Input: part model. Units: mm. Frame: model coordinates. A direction names the side the tool comes from. Coordinates: 2 decimals unless noted, no trailing zeros. Order: outer loops, then holes, each group sorted by start corner. A loop starts at its lowest first (then second) coordinate and runs counter-clockwise, first axis right, second up.
Autodesk Inventor part; units mm, degrees
ref_plane "YZ Plane" through (0, 0, 0) normal (1, 0, 0) x (0, 1, 0)
ref_plane "XZ Plane" through (0, 0, 0) normal (0, 1, 0) x (-1, 0, 0)
ref_plane "XY Plane" through (0, 0, 0) normal (0, 0, 1) x (1, 0, 0)
sketch "Sketch1" plane through (0, 0, 0) normal (0, 0, 1) x (1, 0, 0)
  line L0 (-20, 31) -> (20, 31)
  line L1 (20, 31) -> (20, 0)
  line L2 (-20, 0) -> (-20, 31)
  line L3 (40, 0) -> (40, -20)
  line L4 (40, -20) -> (-40, -20)
  line L5 (-40, -20) -> (-40, 0)
  line L6 (-40, 0) -> (-20, 0)
  line L7 (20, 0) -> (40, 0)
  circle A0 centre (0, 11) radius 9.125
  point P0 (0, 0)
  point P1 (0, 31)
  point P2 (0, -20)
  dimension "d0" = 80
  dimension "d1" = 20
  dimension "d2" = 40
  dimension "d3" = 31
  dimension "d6" = 18.25
  dimension "d7" = 20
extrude "Extrusion1" add sketch "Sketch1" along normal blind 6.5 contours L0 L1 L7 L3 L4 L5 L6 L2 | A0
sketch "Sketch2" plane through (0, 0, 6.5) normal (0, 0, 1) x (1, 0, 0)
  circle A0 centre (0, 11) radius 9.125
  line L0 (20, 31) -> (-20, 31)
  point P0 (0, 0)
  dimension "d8" = 20
  dimension "d9" = 18.25
sketch "Sketch3" plane through (0, 0, 0) normal (0, 0, -1) x (-1, 0, 0)
  line L0 (-20, 31) -> (20, 31)
  line L1 (40, -20) -> (-40, -20)
  line L2 (20, 31) -> (-20, 31)
  line L3 (-20, 31) -> (-20, -20)
  line L4 (-20, -20) -> (20, -20)
  line L5 (20, -20) -> (20, 31)
  point P0 (0, 0)
  point P1 (-20, 5.5)
  point P2 (-20, 0)
extrude "Extrusion2" add sketch "Sketch3" along normal blind 3.5
sketch "Sketch4" plane through (0, 0, -3.5) normal (0, 0, -1) x (-1, 0, 0)
  line L0 (-20, 31) -> (20, 31)
  line L1 (-20, -20) -> (20, -20)
  line L2 (11.85, 31) -> (-11.85, 31)
  line L3 (-11.85, 31) -> (-11.85, -20)
  line L4 (-11.85, -20) -> (11.85, -20)
  line L5 (11.85, -20) -> (11.85, 31)
  point P0 (0, 0)
  point P1 (0, 31)
  dimension "d12" = 23.7
extrude "Extrusion3" add sketch "Sketch4" along normal blind 5
extrude "Extrusion4" cut sketch "Sketch2" against normal up to next
fillet "Fillet1" radius 8 6 edges at (-20, 31, 1.5) (-40, 0, 3.25) (20, 31, 1.5) (-20, 0, 3.25) (40, 0, 3.25) (20, 0, 3.25)
sketch "Sketch5" plane through (0, 0, 0) normal (0, 0, -1) x (-1, 0, 0)
  arc A0 (27.9, -14) -> (32.1, -14) centre (30, -14) ccw
  arc A1 (32.1, -7.88) -> (27.9, -7.88) centre (30, -7.88) ccw
  line L0 (32.1, -7.88) -> (32.1, -14)
  line L1 (27.9, -7.88) -> (27.9, -14)
  line L2 (40, -20) -> (40, -8)
  line L3 (20, -20) -> (40, -20)
  point P0 (0, 0)
  dimension "d18" = 4.2
  dimension "d19" = 6.12
  dimension "d20" = 10
  dimension "d21" = 6
extrude "Extrusion5" cut sketch "Sketch5" against normal up to next
mirror "Mirror1" about plane through (0, 0, 0) normal (1, 0, 0) of "Extrusion5"
properties part number "OldhamCouplerTop"
Item 1: Cut plane B-B on x = 30. Return loops of the section in (y, z).
Response values:
outline: (-20, 0) - (-16.1, 0) - (-16.1, 6.5) - (-20, 6.5) - close; (-5.78, 0) - (0, 0) - (0, 6.5) - (-5.78, 6.5) - close
Item 2: Cut plane C-C on y = 11. Return loops of the section in (x, z) (3 decimals).
Response values:
outline: (-20, -3.5) - (-11.85, -3.5) - (-11.85, -8.5) - (-9.125, -8.5) - (-9.125, 6.5) - (-20, 6.5) - close; (9.125, -8.5) - (11.85, -8.5) - (11.85, -3.5) - (20, -3.5) - (20, 6.5) - (9.125, 6.5) - close
Item 3: Cut plane A-A on z = 4.75. Return loops of the section in (x, y) (3 decimals).
Response values:
outline: (-40, -20) - (40, -20) - (40, -8) arc R8 ccw to (32, 0) - (28, 0) arc R8 cw to (20, 8) - (20, 23) arc R8 ccw to (12, 31) - (-12, 31) arc R8 ccw to (-20, 23) - (-20, 8) arc R8 cw to (-28, 0) - (-32, 0) arc R8 ccw to (-40, -8) - close; hole (-32.1, -14) arc R2.1 ccw to (-27.9, -14) - (-27.9, -7.88) arc R2.1 ccw to (-32.1, -7.88) - close; hole circle Ø18.25 at (0, 11); hole (27.9, -14) arc R2.1 ccw to (32.1, -14) - (32.1, -7.88) arc R2.1 ccw to (27.9, -7.88) - close
Item 4: Draft query along X for faces 4 (the face through (-20, 6, -1)), 5 (the face through (-27.9, -11, 3)), 6 (the face through (-1, -20, 1)), 7 (the face through (30, -16.1, 3.2)). Return one class per face: pulls with the +X half, pulls with the -X half, needs draft (parallel to the pull), parting line crosses it, or undercut.
Response values:
face 4: pulls with the -X half
face 5: undercut
face 6: needs draft
face 7: undercut
Item 5: Cut plane D-D on z = -4.75. Return loops of the section in (x, y) (3 decimals), then the cut area to 3 significant figures.
Response values:
outline: (-11.85, -20) - (11.85, -20) - (11.85, 31) - (-11.85, 31) - close; hole circle Ø18.25 at (0, 11)
area: 947 mm2
Item 6: Access query for faces 1 (the face through (-11.85, 5, -6)), 2 (the face through (27.6, -8.9, 0)), 3 (the face through (29.95, -5.78, 3.2)). Directions: +Z, -Z, +X, -X, +Y, -Y. A direction counts if a zero-diameter tool reaches every point of the face in a straight line with its end or side. Return the directions, or none.
Response values:
face 1: -Z, -X, +Y, -Y
face 2: -Z, +X, +Y, -Y
face 3: +Z, -Z
Item 7: Ray query, probe 1 along X at (y, z) = (-6, 4.5); probe 2 along Y at (x, z) = (0, 2.5) (3 decimals); probe 3 along Z at (x, y) = (-19, 14). Return the intervals inside material, ascending.
Response values:
probe 1: x = -39.75 to -30.94, -29.06 to 29.06, 30.94 to 39.75
probe 2: y = -20 to 1.875, 20.125 to 31
probe 3: z = -3.5 to 6.5
Item 8: Pin query (flat end, axial travel): pin 1 Ø6 at (x, y) = (34.5, 1) entering from -Z; pin 2 Ø2.5 at (y, z) = (1.5, -6.5) entering from +X; pin 3 Ø1 at (y, z) = (16, 4.5) entering from +X. Return the tip coordinate at first contact, or that it passes through.
Response values:
pin 1: stops at z = 0
pin 2: stops at x = 11.85
pin 3: stops at x = 20
